Autodesk Inventor part; units mm, degrees
ref_plane "Work Plane1" through (-126.6696, -48.8832, -9) normal (0, 0, 1) x (1, 0, 0)
ref_plane "YZ Plane" through (0, 0, 0) normal (1, 0, 0) x (0, 1, 0)
ref_plane "XZ Plane" through (0, 0, 0) normal (0, 1, 0) x (-1, 0, 0)
sketch "Sketch1" plane through (0, 0, 0) normal (0, 0, 1) x (1, 0, 0)
  line L0 (58.7032, 31.1168) -> (-11.2968, 31.1168)
  line L1 (-11.2968, 31.1168) -> (-11.2968, -48.8832)
  line L2 (-11.2968, -48.8832) -> (58.7032, -48.8832)
  line L3 (58.7032, -48.8832) -> (58.7032, 31.1168)
  line L4 (53.7032, 16.1168) -> (-6.2968, 16.1168)
  line L5 (-6.2968, 16.1168) -> (-6.2968, -33.8832)
  line L6 (-6.2968, -33.8832) -> (53.7032, -33.8832)
  line L7 (53.7032, -33.8832) -> (53.7032, 16.1168)
  line L8 (58.7032, 31.1168) -> (73.7032, 31.1168)
  line L9 (73.7032, 31.1168) -> (73.7032, 16.1168)
  line L10 (73.7032, 16.1168) -> (58.7032, 16.1168)
  line L11 (58.7032, 16.1168) -> (58.7032, 31.1168)
  point P0 (0, 0)
  dimension "d0" = 70
  dimension "d1" = 80
  dimension "d4" = 60
  dimension "d5" = 50
  dimension "d6" = 15
  dimension "d7" = 5
  dimension "d76" = 15
  dimension "d77" = 15
extrude "Extrusion1" add sketch "Sketch1" along normal blind 7
sketch "Sketch2" plane through (0, 0, 0) normal (0, 0, -1) x (-1, 0, 0)
  line L0 (11.2968, 23.8168) -> (-73.7032, 23.8168)
  line L1 (-73.7032, 23.8168) -> (-73.7032, 18.4168)
  line L2 (-73.7032, 18.4168) -> (11.2968, 18.4168)
  line L3 (11.2968, 18.4168) -> (11.2968, 23.8168)
  line L4 (11.2968, 31.1168) -> (11.2968, -48.8832)
  line L5 (-58.7032, -48.8832) -> (-58.7032, 16.1168)
  line L6 (-73.7032, 16.1168) -> (-73.7032, 31.1168)
  line L7 (-73.7032, 31.1168) -> (11.2968, 31.1168)
  point P0 (0, 0)
  dimension "d9" = 5.4
  dimension "d10" = 0
  dimension "d78" = 0
  dimension "d79" = 7.3
extrude "Extrusion2" add sketch "Sketch2" along normal blind 5.9 draft 9.9 contours L3 L2 L1 L0
ref_plane "Work Plane1" through (-126.6696, -48.8832, -9) normal (0, 0, 1) x (1, 0, 0)
sketch "Sketch3" plane through (0, 0, 0) normal (0, 0, -1) x (-1, 0, 0)
  line L0 (11.2968, -36.3832) -> (-6.7032, -36.3832)
  line L1 (-6.7032, -36.3832) -> (-6.7032, -20.3832)
  line L2 (-6.7032, -20.3832) -> (11.2968, -20.3832)
  line L3 (11.2968, -20.3832) -> (11.2968, -36.3832)
  line L4 (11.2968, -48.8832) -> (-58.7032, -48.8832)
  line L5 (11.2968, 18.4168) -> (11.2968, -48.8832)
  line L6 (-55.7032, -33.3832) -> (-53.7032, -33.3832)
  line L7 (-53.7032, -33.3832) -> (-53.7032, -22.3832)
  line L8 (-53.7032, -22.3832) -> (-55.7032, -22.3832)
  line L9 (-55.7032, -22.3832) -> (-55.7032, -33.3832)
  line L10 (-53.7032, -33.8832) -> (6.2968, -33.8832)
  line L11 (-53.7032, 16.1168) -> (-53.7032, -33.8832)
  point P0 (0, 0)
  point P1 (-54.7032, -33.3832)
  dimension "d14" = 16
  dimension "d15" = 18
  dimension "d16" = 12.5
  dimension "d17" = 0
  dimension "d62" = 11
  dimension "d63" = 0
  dimension "d64" = 2
  dimension "d102" = 0.5
extrude "Extrusion3" add sketch "Sketch3" along normal blind 7.5
sketch "Sketch6" plane through (0, 0, 7) normal (0, 0, 1) x (1, 0, 0)
  line L0 (-6.2968, -20.3832) -> (6.7032, -20.3832)
  line L1 (-11.2968, -48.8832) -> (58.7032, -48.8832)
  line L2 (6.7032, -20.3832) -> (-11.2968, -20.3832)
  line L3 (-11.2968, -20.3832) -> (-11.2968, -48.8832)
  line L4 (-11.2968, -48.8832) -> (6.7032, -48.8832)
  line L5 (6.7032, -48.8832) -> (6.7032, -20.3832)
  point P0 (0, 0)
  point P1 (6.7032, -48.8832)
  point P2 (-6.2968, -20.3832)
extrude "Extrusion6" add sketch "Sketch6" against normal up to surface (7 mm away)
sketch "Sketch9" plane through (-11.2968, -48.8832, 7) normal (-1, 0, 0) x (0, 0, 1)
  circle A0 centre (-10.75, 20.5) radius 3.125
  line L0 (0, 80) -> (0, 0)
  line L1 (-7, 0) -> (0, 0)
  line L2 (-7, 28.5) -> (-7, 65)
  point P0 (-7, 48.8832)
  point P1 (-4, 28.5)
  point P2 (-7, 65)
  dimension "d44" = 6.25
  dimension "d46" = 20.5
  dimension "d65" = 3.75
extrude "Extrusion8" cut sketch "Sketch9" against normal through all
sketch "Sketch10" plane through (0, 0, -7.5) normal (0, 0, -1) x (-1, 0, 0)
  line L0 (1.4968, -23.0332) -> (-3.7032, -23.0332)
  line L1 (-3.7032, -23.0332) -> (-3.7032, -33.7332)
  line L2 (-3.7032, -33.7332) -> (1.4968, -33.7332)
  line L3 (1.4968, -33.7332) -> (1.4968, -23.0332)
  line L4 (11.2968, -20.3832) -> (-6.7032, -20.3832)
  line L5 (-6.7032, -36.3832) -> (11.2968, -36.3832)
  line L6 (-6.7032, -20.3832) -> (-6.7032, -36.3832)
  point P0 (0, 0)
  dimension "d49" = 5.2
  dimension "d50" = 10.7
  dimension "d51" = 2.65
  dimension "d52" = 2.65
  dimension "d53" = 3
extrude "Extrusion9" cut sketch "Sketch10" against normal through all
sketch "Sketch11" plane through (-6.2968, -20.3832, 7) normal (0, 1, 0) x (1, 0, 0)
  circle A0 centre (8, 9.5) radius 1.5
  line L0 (10, 14.5) -> (10, 0)
  line L1 (-5, 14.5) -> (13, 14.5)
  point P0 (6.2968, 7)
  dimension "d56" = 3
  dimension "d57" = 2
  dimension "d58" = 5
extrude "Extrusion10" cut sketch "Sketch11" against normal blind 5
sketch "Sketch12" plane through (0, 0, 0) normal (0, 0, -1) x (-1, 0, 0)
  line L0 (-58.7032, -20.3832) -> (-53.7032, -20.3832)
  line L1 (-53.7032, -20.3832) -> (-53.7032, 12.1168)
  line L2 (-53.7032, 12.1168) -> (-58.7032, 12.1168)
  line L3 (-58.7032, 12.1168) -> (-58.7032, -20.3832)
  line L4 (-53.7032, -22.3832) -> (-55.7032, -22.3832)
  line L5 (-53.7032, 16.1168) -> (-53.7032, -22.3832)
  line L6 (6.2968, 16.1168) -> (-53.7032, 16.1168)
  line L7 (-58.7032, -48.8832) -> (-58.7032, 16.1168)
  line L8 (6.2968, -18.3832) -> (11.2968, -18.3832)
  line L9 (11.2968, -18.3832) -> (11.2968, 11.1168)
  line L10 (11.2968, 11.1168) -> (6.2968, 11.1168)
  line L11 (6.2968, 11.1168) -> (6.2968, -18.3832)
  line L12 (11.2968, -20.3832) -> (-6.7032, -20.3832)
  line L13 (6.2968, -20.3832) -> (6.2968, 16.1168)
  line L14 (11.2968, 18.4168) -> (11.2968, -20.3832)
  point P0 (0, 0)
  point P1 (-58.7032, 18.2168)
  point P2 (-53.7032, -33.8832)
  dimension "d66" = 2
  dimension "d67" = 0
  dimension "d68" = 4
  dimension "d69" = 0
  dimension "d70" = 2
  dimension "d71" = 0
  dimension "d72" = 0
  dimension "d73" = 5
extrude "Extrusion11" cut sketch "Sketch12" against normal blind 2.5 contours L3 L2 L1 L0 | L11 L10 L9 L8
sketch "Sketch13" plane through (0, 0, -7.5) normal (0, 0, -1) x (-1, 0, 0)
  line L0 (-55.7032, -22.3832) -> (-55.7032, -33.3832)
  line L1 (-53.7032, -22.3832) -> (-55.7032, -22.3832)
  line L2 (-55.7032, -33.3832) -> (-53.7032, -33.3832)
  line L3 (-53.7032, -33.3832) -> (-53.7032, -22.3832)
  line L4 (-53.7032, -22.3832) -> (-55.7032, -22.3832)
  line L5 (-55.7032, -22.3832) -> (-55.7032, -33.3832)
  point P0 (0, 0)
extrude "Extrusion12" cut sketch "Sketch13" against normal blind 0.5
chamfer "Chamfer1" distance 3 angle 45 2 edges at (54.7032, -22.3832, -7) (54.7032, -33.3832, -7)
sketch "Sketch14" plane through (0, 0, 7) normal (0, 0, 1) x (1, 0, 0)
  circle A0 centre (-5.2968, 20.1168) radius 1.5
  circle A1 centre (54.7032, 20.1168) radius 1.5
  circle A2 centre (-5.2968, -39.8832) radius 1.5
  circle A3 centre (54.7032, -39.8832) radius 1.5
  line L0 (-11.2968, -48.8832) -> (58.7032, -48.8832)
  line L1 (58.7032, -48.8832) -> (58.7032, 16.1168)
  point P0 (0, 0)
  dimension "d85" = 3
  dimension "d86" = 3
  dimension "d87" = 3
  dimension "d88" = 3
  dimension "d89" = 9
  dimension "d90" = 9
  dimension "d91" = 60
  dimension "d92" = 60
  dimension "d93" = 4
  dimension "d94" = 4
  dimension "d95" = 60
  dimension "d96" = 60
extrude "Extrusion13" cut sketch "Sketch14" against normal through all
chamfer "Chamfer2" distance 7 angle 45 1 edges at (73.7032, 23.6168, 7)
equation "\"d6\" = -0.5 * d5 + 0.5 * d1"
equation "\"d70\" = d66"
equation "\"d90\" = d89"
equation "\"d92\" = d91"
equation "\"d94\" = d93"
equation "\"d96\" = d95"
properties part number "Rail_carriage_y_top_v2"
Verification items for the finished model (mm, model axes). A direction names the side the tool comes from. Coordinates: 2 decimals unless noted, no trailing zeros. Order: outer loops, then holes, each group sorted by start corner. A loop starts at its lowest first (then second) coordinate and runs counter-clockwise, first axis right, second up. Notation, with made-up numbers: (15, 34) -> (36, 34) arc R29 ccw to (36, 62) -> close; hole circle Ø7 at (48.25, 62). An arc over 180 degrees is marked (long way). Answer as CSV lines item,"result". Start each with the question number.
1) Gauge pin test, flat ends, axial feed: pin 1 Ø7.5 at (y, z) = (-8.5, 4.5) entering from +X; pin 2 Ø1.5 at (x, y) = (-8.5, -8) entering from -Z; pin 3 Ø7 at (y, z) = (-2.5, -1.5) entering from -X; pin 4 Ø3.5 at (x, y) = (17, 20.5) entering from -Z. Record the tip position at first contact, or that the pin passes through.
2) Cross-section at C-C, the plane z = -2.5. Give the number of separate pieces and of enclosed holes in the cut face, then the cut area to 3 significant figures.
3) Cross-section at B-B, the plane y = 9. Record the boundary of the cut face in (x, z).
4) Cross-section at A-A, the plane x = 21.5. Record the boundary of the cut face in (y, z).
5) Release check for a two-part mould opening along Z. For faces 6 (the face through (-9, 11.117, 1)), 7 (the face through (54.689, -23.862, -5.479)), 8 (the face through (5.182, -31.434, -4.427)) record: released by +Z, released by -Z, zero draft, split by the parting line, or undercut.
6) Material ranges on L1, parallel to Y at x = -5.5, z = 1.5; L2, parallel to X at y = -32, z = -2.5; L3, parallel to Y at x = 47, z = 1.25, recorded low to high. Write a range as [from, to].
7) Set-up check for faces 1 (the face through (-2, -36.383, -4)), 2 (the face through (58.703, -17, 4)), 3 (the face through (-9, -19, 0)), 4 (the face through (31.81, 17.91, -2.91)), 5 (the face through (1, -23.033, 0)): record each of +Z, -Z, +X, -X, +Y, -Y from which the full face is reachable in a straight line by a thin tool's end or side.
Conclusion:
1,pin 1,"stops at x = 58.7"
1,pin 2,"stops at z = 2.5"
1,pin 3,"passes through"
1,pin 4,"stops at z = -5.9"
2,separate pieces,"6"
2,enclosed holes,"2"
2,area,"686 mm²"
3,outline,"(-11.3, 2.5) -> (-6.3, 2.5) -> (-6.3, 7) -> (-11.3, 7) -> close; (53.7, 2.5) -> (58.7, 2.5) -> (58.7, 7) -> (53.7, 7) -> close"
4,outline,"(-48.88, 0) -> (-33.88, 0) -> (-33.88, 7) -> (-48.88, 7) -> close; (16.12, 0) -> (18.42, 0) -> (17.39, -5.9) -> (24.85, -5.9) -> (23.82, 0) -> (31.12, 0) -> (31.12, 7) -> (16.12, 7) -> close"
5,face 6,"zero draft"
5,face 7,"released by -Z"
5,face 8,"undercut"
6,L1,"y = [-48.88, -41.37], [-38.4, -20.38], [16.12, 18.63], [21.6, 31.12]"
6,L2,"x = [-11.3, -1.5], [3.7, 6.7], [53.7, 55.7]"
6,L3,"y = [-48.88, -33.88], [16.12, 31.12]"
7,face 1,"-Z, +X, -X, -Y"
7,face 2,"+Z, -Z, +X, -Y"
7,face 3,"-Z, +X, -X"
7,face 4,"+X, -X"
7,face 5,"+Z, -Z"
